```python
from build123d import *

# Parameters (mm, degrees)
SKETCH1_R                = 29
SKETCH1_R_2              = 2.5
BOSS_EXTRUDE1_DEPTH      = 11.34
SKETCH2_R                = 4
SKETCH2_R_2              = 2.5
BOSS_EXTRUDE2_DEPTH      = 14.5
SKETCH3_R                = 5
SKETCH3_R_2              = 4
BOSS_EXTRUDE3_DEPTH      = 1.5
BOSS_EXTRUDE4_DEPTH      = 14.5
FILLET2_R                = 0.5
FILLET5_R                = 1.5
CIRPATTERN1_COUNT        = 3
FILLET2_OF_CIRPATTERN1_R = 0.5
FILLET5_OF_CIRPATTERN1_R = 1.5
SKETCH5_R                = 1.5
CUT_EXTRUDE1_DEPTH       = 49.473761975
SKETCH6_R                = 2.75
CUT_EXTRUDE2_DEPTH       = 3
SKETCH7_R                = 4.25
CUT_EXTRUDE3_DEPTH       = 5
CIRPATTERN2_COUNT        = 3
CHAMFER1_SIZE            = 0.5
SKETCH9_R                = 8
CUT_EXTRUDE4_DEPTH       = 44.5
BOSS_EXTRUDE7_START      = -7.34
SKETCH10_R               = 8
SKETCH10_R_2             = 6.5
BOSS_EXTRUDE7_DEPTH      = 7.34
CHAMFER2_SIZE            = 0.5
BOSS_EXTRUDE8_START      = -1.5
SKETCH11_R               = 30.5
SKETCH11_R_2             = 29
BOSS_EXTRUDE8_DEPTH      = 1.5


with BuildPart() as part:
    # Sketch1 → Boss-Extrude1 (new body)
    with BuildSketch(Plane.XY):
        with Locations(Location((0, 0, 0), (0, 0, 180))):
            Circle(SKETCH1_R)
        with Locations(Location((0, 24, 0), (0, 0, 180))):
            Circle(SKETCH1_R_2, mode=Mode.SUBTRACT)
        with Locations(Location((20.784609691, -12, 0), (0, 0, 180))):
            Circle(SKETCH1_R_2, mode=Mode.SUBTRACT)
        with Locations(Location((-20.784609691, -12, 0), (0, 0, 180))):
            Circle(SKETCH1_R_2, mode=Mode.SUBTRACT)
    extrude(amount=BOSS_EXTRUDE1_DEPTH)

    # Sketch2 → Boss-Extrude2 (add)
    with BuildSketch(Plane.XY.offset(11.34)):
        with Locations(Location((0, 24, 0), (0, 0, 180))):
            Circle(SKETCH2_R)
        with Locations(Location((0, 24, 0), (0, 0, 180))):
            Circle(SKETCH2_R_2, mode=Mode.SUBTRACT)
    boss_extrude2 = extrude(amount=BOSS_EXTRUDE2_DEPTH)

    # Sketch3 → Boss-Extrude3 (add)
    with BuildSketch(Plane.XY.offset(11.34)):
        with Locations(Location((0, 24, 0), (0, 0, 90))):
            Circle(SKETCH3_R)
        with Locations(Location((0, 24, 0), (0, 0, 180))):
            Circle(SKETCH3_R_2, mode=Mode.SUBTRACT)
    boss_extrude3 = extrude(amount=BOSS_EXTRUDE3_DEPTH)

    # Sketch4 → Boss-Extrude4 (add)
    with BuildSketch(Plane.XY.offset(11.34)):
        with BuildLine():
            ThreePointArc((-9.243861456, 9.140625), (-15.08397544, 15.127363136), (-17.478886538, 23.140625))
            ThreePointArc((-17.478886538, 23.140625), (-25.11473671, 14.5), (-28.779812378, 3.566847272))
            ThreePointArc((-28.779812378, 3.566847272), (-20.642668488, 5.499424353), (-12.537944184, 3.43510635))
            ThreePointArc((-12.537944184, 3.43510635), (-11.258330249, 6.5), (-9.243861456, 9.140625))
        make_face()
    boss_extrude4 = extrude(amount=BOSS_EXTRUDE4_DEPTH)

    # Fillet2
    fillet2_edges = [part.edges().sort_by_distance(p)[0] for p in [
        (0, 19, 12.84),
    ]]
    fillet(fillet2_edges, radius=FILLET2_R)

    # Fillet5
    # the kernel refuses this fillet: 1.5 mm, written as the material it takes off along each edge
    with BuildSketch(Plane(origin=(-17.478886538, 23.140625, 11.34), x_dir=(0.12399934101480344, -0.9922823002693812, 0), z_dir=(0, 0, 1))) as fillet5_piece_1:
        with BuildLine():
            CenterArc((2.741938005, -1.495761572), FILLET5_R, 94.30820856, 121.194344996)
            ThreePointArc((1.52080355, -2.36687043), (0.731683032, -1.201888091), (0, 0))
            ThreePointArc((0, 0), (1.314627811, -0.049448326), (2.629255621, 0))
        make_face()
    extrude(amount=21.53336649, mode=Mode.SUBTRACT)
    with BuildSketch(Plane(origin=(-28.779812378, 3.566847272, 11.34), x_dir=(0.9213413502663426, 0.3887545707633453, 0), z_dir=(0, 0, 1))) as fillet5_piece_2:
        with BuildLine():
            CenterArc((2.741938005, 1.495761572), FILLET5_R, 144.497446444, 121.194344996)
            ThreePointArc((1.52080355, 2.36687043), (0.731683032, 1.201888091), (0, 0))
            ThreePointArc((0, 0), (1.314627811, 0.049448326), (2.629255621, 0))
        make_face()
    extrude(amount=21.53336649, mode=Mode.SUBTRACT)
    with BuildSketch(Plane(origin=(-12.537944184, 3.43510635, 11.34), x_dir=(-0.9027827871570022, 0.430096778891722, 0), z_dir=(0, 0, 1))) as fillet5_piece_3:
        with BuildLine():
            CenterArc((1.681832709, -1.498406794), FILLET5_R, 92.640987591, 90.493935252)
            ThreePointArc((0.184077424, -1.580437939), (0.116240905, -0.787400081), (0, 0))
            ThreePointArc((0, 0), (0.806358148, -0.018587399), (1.612716296, 0))
        make_face()
    extrude(amount=18.53179074, mode=Mode.SUBTRACT)
    with BuildSketch(Plane(origin=(-9.243861456, 9.140625, 11.34), x_dir=(-0.6582920213979585, -0.7527626548679136, 0), z_dir=(0, 0, 1))) as fillet5_piece_4:
        with BuildLine():
            CenterArc((1.682917286, -1.497188561), FILLET5_R, 93.508521646, 90.493935252)
            ThreePointArc((0.186575699, -1.601887437), (0.11175044, -0.798793336), (0, 0))
            ThreePointArc((0, 0), (0.795560899, -0.024365801), (1.591121798, 0))
        make_face()
    extrude(amount=18.53179074, mode=Mode.SUBTRACT)

    # CirPattern1: Boss-Extrude2, Boss-Extrude3, Boss-Extrude4 ×3 about axis
    cirpattern1_axis = Axis((0, 0, 0), (0, 0, 1))
    add([boss_extrude2.rotate(cirpattern1_axis, i * 360 / CIRPATTERN1_COUNT) for i in range(1, CIRPATTERN1_COUNT)])
    add([boss_extrude3.rotate(cirpattern1_axis, i * 360 / CIRPATTERN1_COUNT) for i in range(1, CIRPATTERN1_COUNT)])
    add([boss_extrude4.rotate(cirpattern1_axis, i * 360 / CIRPATTERN1_COUNT) for i in range(1, CIRPATTERN1_COUNT)])

    # Fillet2 of CirPattern1
    fillet2_of_cirpattern1_edges = [part.edges().sort_by_distance(p)[0] for p in [
        (-16.454482672, -9.5, 12.84),
        (16.454482672, -9.5, 12.84),
    ]]
    fillet(fillet2_of_cirpattern1_edges, radius=FILLET2_OF_CIRPATTERN1_R)

    # Fillet5 of CirPattern1
    # the kernel refuses this fillet: 1.5 mm, written as the material it takes off along each edge
    with BuildSketch(Plane(origin=(-11.30092584, -26.707472272, 11.34), x_dir=(0.9387654185354608, -0.3445569458913013, 0), z_dir=(0, 0, 1))) as fillet5_of_cirpattern1_piece_1:
        with BuildLine():
            CenterArc((2.740587632, 1.498234339), FILLET5_OF_CIRPATTERN1_R, 151.58593368, 121.194344996)
            ThreePointArc((1.421289964, 2.211994566), (0.752245893, 1.079267128), (0, 0))
            ThreePointArc((0, 0), (1.406673298, -0.034136121), (2.813346596, 0))
        make_face()
    extrude(amount=21.53336649, mode=Mode.SUBTRACT)
    with BuildSketch(Plane(origin=(11.30092584, -26.707472272, 11.34), x_dir=(-0.9387654185354388, -0.3445569458913611, 0), z_dir=(0, 0, 1))) as fillet5_of_cirpattern1_piece_2:
        with BuildLine():
            CenterArc((2.740587632, -1.498234339), FILLET5_OF_CIRPATTERN1_R, 87.219721325, 121.194344996)
            ThreePointArc((1.421289964, -2.211994566), (0.752245893, -1.079267128), (0, 0))
            ThreePointArc((0, 0), (1.406673298, 0.034136121), (2.813346596, 0))
        make_face()
    extrude(amount=21.53336649, mode=Mode.SUBTRACT)
    with BuildSketch(Plane(origin=(3.294082729, -12.57573135, 11.34), x_dir=(0.07891665697240977, -0.9968812172231449, 0), z_dir=(0, 0, 1)), Plane(origin=(9.243861456, 9.140625, 11.34), x_dir=(0.823866130184591, 0.5667844383314229, 0), z_dir=(0, 0, 1))) as fillet5_of_cirpattern1_piece_3:
        with BuildLine():
            CenterArc((1.681832709, -1.498406794), FILLET5_OF_CIRPATTERN1_R, 92.640987591, 90.493935252)
            ThreePointArc((0.184077424, -1.580437939), (0.116240905, -0.787400081), (0, 0))
            ThreePointArc((0, 0), (0.806358148, -0.018587399), (1.612716296, 0))
        make_face()
    extrude(amount=18.53179074, mode=Mode.SUBTRACT)
    with BuildSketch(Plane(origin=(-3.294082729, -12.57573135, 11.34), x_dir=(0.9810575928348104, -0.19371628620528378, 0), z_dir=(0, 0, 1)), Plane(origin=(12.537944184, 3.43510635, 11.34), x_dir=(-0.3227655714368486, 0.9464789410731993, 0), z_dir=(0, 0, 1))) as fillet5_of_cirpattern1_piece_4:
        with BuildLine():
            CenterArc((1.682917286, -1.497188561), FILLET5_OF_CIRPATTERN1_R, 93.508521646, 90.493935252)
            ThreePointArc((0.186575699, -1.601887437), (0.11175044, -0.798793336), (0, 0))
            ThreePointArc((0, 0), (0.795560899, -0.024365801), (1.591121798, 0))
        make_face()
    extrude(amount=18.53179074, mode=Mode.SUBTRACT)
    with BuildSketch(Plane(origin=(28.779812378, 3.566847272, 11.34), x_dir=(-0.9213413502663421, 0.38875457076334596, 0), z_dir=(0, 0, 1))) as fillet5_of_cirpattern1_piece_5:
        with BuildLine():
            CenterArc((2.741938005, -1.495761572), FILLET5_OF_CIRPATTERN1_R, 94.30820856, 121.194344996)
            ThreePointArc((1.52080355, -2.36687043), (0.731683032, -1.201888091), (0, 0))
            ThreePointArc((0, 0), (1.314627811, -0.049448326), (2.629255621, 0))
        make_face()
    extrude(amount=21.53336649, mode=Mode.SUBTRACT)
    with BuildSketch(Plane(origin=(17.478886538, 23.140625, 11.34), x_dir=(-0.12399934101479214, -0.9922823002693827, 0), z_dir=(0, 0, 1))) as fillet5_of_cirpattern1_piece_6:
        with BuildLine():
            CenterArc((2.741938005, 1.495761572), FILLET5_OF_CIRPATTERN1_R, 144.497446444, 121.194344996)
            ThreePointArc((1.52080355, 2.36687043), (0.731683032, 1.201888091), (0, 0))
            ThreePointArc((0, 0), (1.314627811, 0.049448326), (2.629255621, 0))
        make_face()
    extrude(amount=21.53336649, mode=Mode.SUBTRACT)

    # Sketch5 → Cut-Extrude1 (cut, through all)
    with BuildSketch(Plane.XY.offset(25.84)):
        with Locations((-21.650635095, 12.5)):
            Circle(SKETCH5_R)
    cut_extrude1 = extrude(amount=-CUT_EXTRUDE1_DEPTH, mode=Mode.SUBTRACT)

    # Sketch6 → Cut-Extrude2 (cut)
    with BuildSketch(Plane(origin=(0, 0, 0), x_dir=(-1, 0, 0), z_dir=(0, 0, -1))):
        with Locations((21.650635095, 12.5)):
            Circle(SKETCH6_R)
    cut_extrude2 = extrude(amount=-CUT_EXTRUDE2_DEPTH, mode=Mode.SUBTRACT)

    # Sketch7 → Cut-Extrude3 (cut)
    with BuildSketch(Plane(origin=(0, 0, 0), x_dir=(-1, 0, 0), z_dir=(0, 0, -1))):
        with Locations((0, 24)):
            Circle(SKETCH7_R)
    cut_extrude3 = extrude(amount=-CUT_EXTRUDE3_DEPTH, mode=Mode.SUBTRACT)

    # CirPattern2: Cut-Extrude1, Cut-Extrude2, Cut-Extrude3 ×3 about axis
    cirpattern2_axis = Axis((0, 0, 0), (0, 0, 1))
    add([cut_extrude1.rotate(cirpattern2_axis, i * 360 / CIRPATTERN2_COUNT) for i in range(1, CIRPATTERN2_COUNT)], mode=Mode.SUBTRACT)
    add([cut_extrude2.rotate(cirpattern2_axis, i * 360 / CIRPATTERN2_COUNT) for i in range(1, CIRPATTERN2_COUNT)], mode=Mode.SUBTRACT)
    add([cut_extrude3.rotate(cirpattern2_axis, i * 360 / CIRPATTERN2_COUNT) for i in range(1, CIRPATTERN2_COUNT)], mode=Mode.SUBTRACT)

    # Chamfer1
    chamfer1_edges = [part.edges().sort_by_distance(p)[0] for p in [
        (29, 0, 0),
    ]]
    chamfer(chamfer1_edges, length=CHAMFER1_SIZE)

    # Sketch9 → Cut-Extrude4 (cut, through all)
    with BuildSketch(Plane.XY.offset(11.34)):
        Circle(SKETCH9_R)
    extrude(amount=-CUT_EXTRUDE4_DEPTH, mode=Mode.SUBTRACT)

    # Sketch10 → Boss-Extrude7 (add)
    with BuildSketch(Plane(origin=(0, 0, 0), x_dir=(-1, 0, 0), z_dir=(0, 0, -1)).offset(BOSS_EXTRUDE7_START)):
        with Locations(Location((0, 0, 0), (0, 0, 180))):
            Circle(SKETCH10_R)
        Circle(SKETCH10_R_2, mode=Mode.SUBTRACT)
    extrude(amount=BOSS_EXTRUDE7_DEPTH)

    # Chamfer2
    chamfer2_edges = [part.edges().sort_by_distance(p)[0] for p in [
        (-8, 0, 11.34),
    ]]
    chamfer(chamfer2_edges, length=CHAMFER2_SIZE)

    # Sketch11 → Boss-Extrude8 (add)
    with BuildSketch(Plane.XY.offset(11.34).offset(BOSS_EXTRUDE8_START)):
        Circle(SKETCH11_R)
        with Locations(Location((0, 0, 0), (0, 0, 180))):
            Circle(SKETCH11_R_2, mode=Mode.SUBTRACT)
    extrude(amount=BOSS_EXTRUDE8_DEPTH)


solid = part.part
```
Geometry check sheet. Reference: the model listing, model coordinates, mm. A direction names the side the tool comes from. Coordinates: 2 decimals unless noted, no trailing zeros. Order: outer loops, then holes, each group sorted by start corner. A loop starts at its lowest first (then second) coordinate and runs counter-clockwise, first axis right, second up. Notation, with made-up numbers: (29, 72) - (36, 72) arc R21 cw to (36, 106) - close; hole circle Ø4 at (3.25, 57). An arc over 180 degrees is marked (long way). Answer as a JSON object with one key per item and string values. Group by question number.
Item 1: Sectioned sample at A-A, the plane y = 0. Record the cut outline in (x, z).
Item 2: Sectioned sample at B-B, the plane z = 23.25. Give the number of separate pieces and of enclosed holes in the cut face, and give its area (3 significant figures).
Item 3: Scan lines: probe 1 along Y at (x, z) = (23, 1.5); probe 2 along Y at (x, z) = (20.5, 16.75); probe 3 along X at (y, z) = (26, 20.5). Record each from-to range of solid material in increasing order.
Item 4: Draft check along X on faces 1 (the face through (-19, 11, 25.84)), 2 (the face through (-24.204, -18.559, 10.58)), 3 (the face through (-2, 22, 5)), 4 (the face through (18.63, -15.37, 19.25)). Enter one of: +X half, -X half, draft (parallel to the pull), parting line (faces both ways), or undercut.
Item 5: Depth check by flat-ended pin: pin 1 Ø6 at (x, y) = (-0.5, -10) entering from -Z; pin 2 Ø4 at (x, y) = (-0.5, 23) entering from -Z; pin 3 Ø1.5 at (y, z) = (-12.5, 21) entering from -X; pin 4 Ø1 at (x, z) = (3, 4.5) entering from +Y. Enter the tip coordinate at first touch or a pass-through.
Item 6: Tool access check on faces 5 (the face through (-1.27, -27.44, 1.48)), 6 (the face through (0, -29, 18)), 7 (the face through (3, 21, 12.84)), 8 (the face through (18.97, -10.28, 15.27)). Record the directions out of +Z, -Z, +X, -X, +Y, -Y that give a thin tool (end or side, any length) a straight path to the whole face; none if there is none.
Resolved:
{
 "1": {"outline": "(-30.5, 9.84) - (-29, 9.84) - (-29, 0.5) - (-28.5, 0) - (-6.5, 0) - (-6.5, 7.34) - (-8, 7.34) - (-8, 10.84) - (-8.5, 11.34) - (-30.5, 11.34) - close; (6.5, 0) - (28.5, 0) - (29, 0.5) - (29, 9.84) - (30.5, 9.84) - (30.5, 11.34) - (8.5, 11.34) - (8, 10.84) - (8, 7.34) - (6.5, 7.34) - close"},
 "2": {"separate pieces": "6", "enclosed holes": "6", "area": "643 mm^2"},
 "3": {"probe 1": "-17.66 to -15.63, -8.37 to 10.1, 14.9 to 17.66", "probe 2": "-15.99 to -14.48, -9.52 to -8.01, 5.5 to 11.54, 13.46 to 20.51", "probe 3": "-3.46 to -1.5, 1.5 to 3.46"},
 "4": {"face 1": "draft", "face 2": "parting line", "face 3": "undercut", "face 4": "undercut"},
 "5": {"pin 1": "z = 0", "pin 2": "z = 5", "pin 3": "x = -24.78", "pin 4": "y = 28.89"},
 "6": {"face 5": "-Z", "face 6": "+Z, -Y", "face 7": "+Z", "face 8": "+Z, -Z"}
}
